Geometry: final body of the model. Coordinates: model frame, mm. Face numbers are marked on the shaded views. Round coordinates to 2 decimals unless told otherwise and drop trailing zeros. Loops run counter-clockwise (first coordinate to the right, second up) from the corner with the lowest first, then second, coordinate; pieces in that order, holes last. Notation, with made-up numbers: (56.5, 80) - (73.5, 80) arc R8 cw to (73.5, 90) - close; hole circle Ø7 at (39.5, 53). An arc over 180 degrees is marked (long way). Write item = value, one per line. Start each with the question number.
Item 1: Section C-C (x = 38). Return loops of the section in (y, z).
Item 2: Section B-B (x = 25.4). Return loops of the section in (y, z), plus the area to 3 significant figures.
Item 3: Section A-A (z = 12.7). Return loops of the section in (x, y) (3 decimals), plus the area to 3 significant figures.
Item 4: Section D-D (y = 8.25). Count the separate pieces of the cut face and the enclosed holes in it, plus the area to 3 significant figures.
Item 5: Line query: line 1 (X direction, y = -2.5, z = -13); line 2 (Z direction, x = 38.1, y = 4) (3 decimals); line 3 (Z direction, x = 25.4, y = -11.7). Output: solid intervals per line, ascending. Write a range as from..to.
Item 6: Draft query along X for the marked faces 1, 2, 3 and 4. Return one class per face: pulls with the +X half, pulls with the -X half, needs draft (parallel to the pull), parting line crosses it, or undercut.
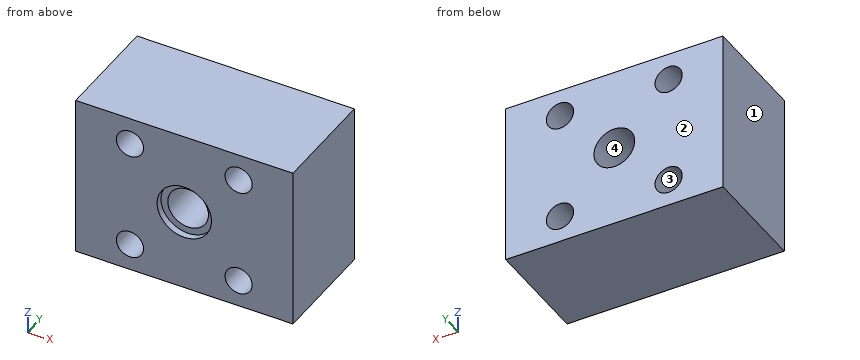
from build123d import *

# Parameters (mm, degrees)
F0_W     = 25.4
F0_H     = 38.1
F1_DEPTH = 50.8
F2_R     = 3.175
F3_DEPTH = 25.4
F4_R     = 6.35
F5_DEPTH = 1.5875
F6_R     = 4.7625
F7_DEPTH = 25.4


with BuildPart() as f1:
    # F0 (on Right) → F1 (new body)
    with BuildSketch(Plane.YZ):
        Rectangle(F0_W, F0_H)
    extrude(amount=F1_DEPTH)

    # F2 (on face) → F3 (cut)
    with BuildSketch(Plane.XZ.offset(12.7)):
        with Locations((12.7, 12.7)):
            Circle(F2_R)
        with Locations((38.1, -12.7)):
            Circle(F2_R)
        with Locations((38.1, 12.7)):
            Circle(F2_R)
        with Locations((12.7, -12.7)):
            Circle(F2_R)
    extrude(amount=-F3_DEPTH, mode=Mode.SUBTRACT)

    # F4 (on face) → F5 (cut)
    with BuildSketch(Plane.XZ.offset(12.7)):
        with Locations((25.4, 0)):
            Circle(F4_R)
    extrude(amount=-F5_DEPTH, mode=Mode.SUBTRACT)

    # F6 (on face) → F7 (cut)
    with BuildSketch(Plane(origin=(0, 12.7, 0), x_dir=(-1, 0, 0), z_dir=(0, 1, 0))):
        with Locations((-25.4, 0)):
            Circle(F6_R)
    extrude(amount=-F7_DEPTH, mode=Mode.SUBTRACT)


solid = f1.part
Taken from the geometry:
q1.outline = (-12.7, -19.05) - (12.7, -19.05) - (12.7, -15.87) - (-12.7, -15.87) - close; (-12.7, -9.53) - (12.7, -9.53) - (12.7, 9.53) - (-12.7, 9.53) - close; (-12.7, 15.87) - (12.7, 15.87) - (12.7, 19.05) - (-12.7, 19.05) - close
q2.outline = (-12.7, -19.05) - (12.7, -19.05) - (12.7, -4.76) - (-11.11, -4.76) - (-11.11, -6.35) - (-12.7, -6.35) - close; (-12.7, 6.35) - (-11.11, 6.35) - (-11.11, 4.76) - (12.7, 4.76) - (12.7, 19.05) - (-12.7, 19.05) - close
q2.area = 721 mm^2
q3.outline = (0, -12.7) - (9.525, -12.7) - (9.525, 12.7) - (0, 12.7) - close; (15.875, -12.7) - (34.925, -12.7) - (34.925, 12.7) - (15.875, 12.7) - close; (41.275, -12.7) - (50.8, -12.7) - (50.8, 12.7) - (41.275, 12.7) - close
q3.area = 968 mm^2
q4.separate_pieces = 1
q4.enclosed_holes = 5
q4.area = 1,740 mm^2
q5.line_1 = 0..9.54, 15.86..34.94, 41.26..50.8
q5.line_2 = -19.05..-15.875, -9.525..9.525, 15.875..19.05
q5.line_3 = -19.05..-6.35, 6.35..19.05
q6.face_1 = pulls with the -X half
q6.face_2 = needs draft
q6.face_3 = undercut
q6.face_4 = undercut
